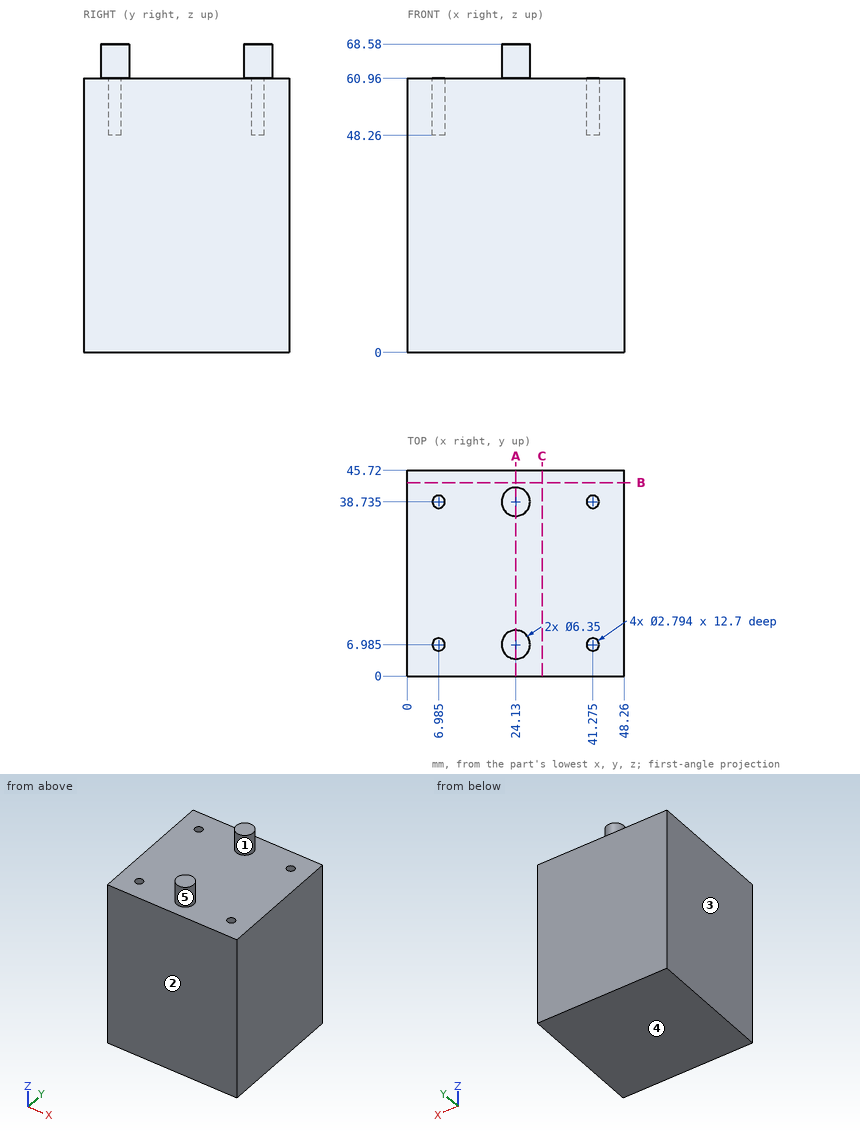
Drawing for the job (mm, zero at the part's lowest x, y, z). A direction names the side the tool comes from. Round coordinates to 2 decimals unless told otherwise and drop trailing zeros. Write each loop counter-clockwise with the first axis right and the second up, starting at its lowest first coordinate (ties: lowest second). Pieces come first, ordered by that corner, then holes. Notation, with made-up numbers: (3.25, 20) - (19.25, 20) arc R19 cw to (19.25, 36) - close; hole circle Ø5 at (-25, -37.5). An arc over 180 degrees is marked (long way). Return JSON: item names as keys, results as strings. Group by question number.
Item 1: Flat gauge pins, fed straight in: pin 1 Ø1.4 at (x, y) = (6.5, 7) entering from +Z; pin 2 Ø1 at (x, z) = (25.5, 13.5) entering from -Y; pin 3 Ø4 at (x, y) = (37.5, 11) entering from +Z. Where does each tip first touch, or does it go through?
Item 2: Probe probe 1 along Z at (x, y) = (12, 11.5); probe 2 along Y at (x, z) = (22.5, 62.5); probe 3 along Y at (x, z) = (24.5, 63). List the from-to ranges inside material, lowest first.
Item 3: Mould opens along X. For the marked faces 3, 4 and 5 say: +X half, -X half, draft (parallel to the pull), parting line (faces both ways), or undercut.
Item 4: Band-saw the part on C-C on x = 30. List the corners of the cut face in (y, z), plus the area to 3 significant figures.
Item 5: Band-saw the part on A-A on x = 24.13. List the corners of the cut face in (y, z).
Item 6: Band-saw the part on B-B on y = 43. List the corners of the cut face in (x, z), plus the area to 3 significant figures.
Item 7: 3-axis set-ups, long thin cutter, end or side, ignore diameter. For the marked faces 1 and 2: which of +Z, -Z, +X, -X, +Y, -Y reach the whole face in a straight line?
Resolved:
{
 "1": {"pin 1": "stops at z = 48.26", "pin 2": "stops at y = 0", "pin 3": "stops at z = 60.96"},
 "2": {"probe 1": "z = 0 to 60.96", "probe 2": "y = 4.26 to 9.71, 36.01 to 41.46", "probe 3": "y = 3.83 to 10.14, 35.58 to 41.89"},
 "3": {"face 3": "-X half", "face 4": "draft", "face 5": "parting line"},
 "4": {"outline": "(0, 0) - (45.72, 0) - (45.72, 60.96) - (0, 60.96) - close", "area": "2,790 mm²"},
 "5": {"outline": "(0, 0) - (45.72, 0) - (45.72, 60.96) - (41.91, 60.96) - (41.91, 68.58) - (35.56, 68.58) - (35.56, 60.96) - (10.16, 60.96) - (10.16, 68.58) - (3.81, 68.58) - (3.81, 60.96) - (0, 60.96) - close"},
 "6": {"outline": "(0, 0) - (48.26, 0) - (48.26, 60.96) - (0, 60.96) - close", "area": "2,940 mm²"},
 "7": {"face 1": "+Z", "face 2": "+Z, -Z, +X, -X, -Y"}
}
